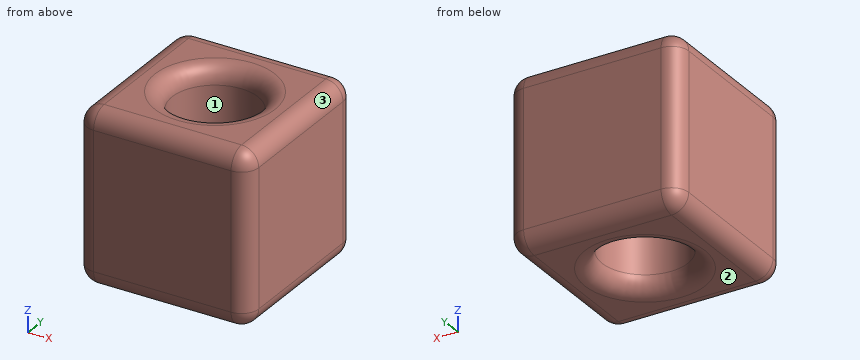
```python
from build123d import *

# Parameters (mm, degrees)
SKETCH2_W           = 100
SKETCH2_H           = 100
BOSS_EXTRUDE1_DEPTH = 100
SKETCH3_R           = 25
CUT_EXTRUDE1_DEPTH  = 100
FILLET1_R           = 10
FILLET2_R           = 10
FILLET3_R           = 10
FILLET4_R           = 10


with BuildPart() as part:
    # Sketch2 → Boss-Extrude1 (new body)
    with BuildSketch(Plane(origin=(0, 0, 0), x_dir=(1, 0, 0), z_dir=(0, 1, 0))):
        with Locations((50, 50)):
            Rectangle(SKETCH2_W, SKETCH2_H)
    extrude(amount=BOSS_EXTRUDE1_DEPTH)

    # Sketch3 → Cut-Extrude1 (cut)
    with BuildSketch(Plane.XY):
        with Locations((50, 50)):
            Circle(SKETCH3_R)
    extrude(amount=-CUT_EXTRUDE1_DEPTH, mode=Mode.SUBTRACT)

    # Fillet1
    fillet1_edges = [part.edges().sort_by_distance(p)[0] for p in [
        (25, 50, 0),
        (50, 0, 0),
        (100, 50, 0),
        (0, 50, 0),
        (50, 100, 0),
    ]]
    fillet(fillet1_edges, radius=FILLET1_R)

    # Fillet2
    fillet2_edges = [part.edges().sort_by_distance(p)[0] for p in [
        (25, 50, -100),
        (50, 100, -100),
        (50, 0, -100),
        (0, 50, -100),
        (100, 50, -100),
    ]]
    fillet(fillet2_edges, radius=FILLET2_R)

    # Fillet3
    # the kernel refuses this fillet: 10 mm, written as the material it takes off along each edge
    with BuildSketch(Plane(origin=(90, 90, -10), x_dir=(1, 0, 0), z_dir=(0, 1, 0))) as fillet3_piece_1_section:
        Polygon((0, 0), (FILLET3_R, 0), (FILLET3_R, -FILLET3_R), (0, -FILLET3_R), align=None)
    fillet3_piece_1 = extrude(amount=FILLET3_R, mode=Mode.PRIVATE)
    fillet3_piece_1 = fillet3_piece_1 - Plane(origin=(90, 90, -10), x_dir=(-0.7071067811865475, 0, -0.7071067811865475), z_dir=(0, 1, 0)) * Sphere(FILLET3_R, mode=Mode.PRIVATE)
    add(fillet3_piece_1, mode=Mode.SUBTRACT)
    with BuildSketch(Plane(origin=(90, 10, -10), x_dir=(0, -1, 0), z_dir=(1, 0, 0))) as fillet3_piece_2_section:
        Polygon((0, 0), (FILLET3_R, 0), (FILLET3_R, -FILLET3_R), (0, -FILLET3_R), align=None)
    fillet3_piece_2 = extrude(amount=FILLET3_R, mode=Mode.PRIVATE)
    fillet3_piece_2 = fillet3_piece_2 - Plane(origin=(90, 10, -10), x_dir=(0, 0.7071067811865475, -0.7071067811865475), z_dir=(1, 0, 0)) * Sphere(FILLET3_R, mode=Mode.PRIVATE)
    add(fillet3_piece_2, mode=Mode.SUBTRACT)
    with BuildSketch(Plane(origin=(90, 90, -90), x_dir=(1, 0, 0), z_dir=(0, 1, 0))) as fillet3_piece_3_section:
        Polygon((0, 0), (FILLET3_R, 0), (FILLET3_R, FILLET3_R), (0, FILLET3_R), align=None)
    fillet3_piece_3 = extrude(amount=FILLET3_R, mode=Mode.PRIVATE)
    fillet3_piece_3 = fillet3_piece_3 - Plane(origin=(90, 90, -90), x_dir=(-0.7071067811865475, 0, 0.7071067811865475), z_dir=(0, 1, 0)) * Sphere(FILLET3_R, mode=Mode.PRIVATE)
    add(fillet3_piece_3, mode=Mode.SUBTRACT)
    with BuildSketch(Plane(origin=(90, 10, -90), x_dir=(0, -1, 0), z_dir=(1, 0, 0))) as fillet3_piece_4_section:
        Polygon((0, 0), (FILLET3_R, 0), (FILLET3_R, FILLET3_R), (0, FILLET3_R), align=None)
    fillet3_piece_4 = extrude(amount=FILLET3_R, mode=Mode.PRIVATE)
    fillet3_piece_4 = fillet3_piece_4 - Plane(origin=(90, 10, -90), x_dir=(0, 0.7071067811865475, 0.7071067811865475), z_dir=(1, 0, 0)) * Sphere(FILLET3_R, mode=Mode.PRIVATE)
    add(fillet3_piece_4, mode=Mode.SUBTRACT)
    with BuildSketch(Plane(origin=(100, 100, -10), x_dir=(-1, 0, 0), z_dir=(0, 0, -1)), Plane(origin=(100, 0, -10), x_dir=(0, 1, 0), z_dir=(0, 0, -1))) as fillet3_piece_5:
        with BuildLine():
            CenterArc((FILLET3_R, -FILLET3_R), FILLET3_R, 90, 90)
            Line((0, -FILLET3_R), (0, 0))
            Line((0, 0), (FILLET3_R, 0))
        make_face()
    extrude(amount=80, mode=Mode.SUBTRACT)

    # Fillet4
    # the kernel refuses this fillet: 10 mm, written as the material it takes off along each edge
    with BuildSketch(Plane(origin=(10, 90, -10), x_dir=(-1, 0, 0), z_dir=(0, 1, 0))) as fillet4_piece_1_section:
        Polygon((0, 0), (FILLET4_R, 0), (FILLET4_R, FILLET4_R), (0, FILLET4_R), align=None)
    fillet4_piece_1 = extrude(amount=FILLET4_R, mode=Mode.PRIVATE)
    fillet4_piece_1 = fillet4_piece_1 - Plane(origin=(10, 90, -10), x_dir=(0.7071067811865475, 0, -0.7071067811865475), z_dir=(0, 1, 0)) * Sphere(FILLET4_R, mode=Mode.PRIVATE)
    add(fillet4_piece_1, mode=Mode.SUBTRACT)
    with BuildSketch(Plane(origin=(10, 10, -10), x_dir=(0, -1, 0), z_dir=(-1, 0, 0))) as fillet4_piece_2_section:
        Polygon((0, 0), (FILLET4_R, 0), (FILLET4_R, FILLET4_R), (0, FILLET4_R), align=None)
    fillet4_piece_2 = extrude(amount=FILLET4_R, mode=Mode.PRIVATE)
    fillet4_piece_2 = fillet4_piece_2 - Plane(origin=(10, 10, -10), x_dir=(0, 0.7071067811865475, -0.7071067811865475), z_dir=(-1, 0, 0)) * Sphere(FILLET4_R, mode=Mode.PRIVATE)
    add(fillet4_piece_2, mode=Mode.SUBTRACT)
    with BuildSketch(Plane(origin=(10, 90, -90), x_dir=(-1, 0, 0), z_dir=(0, 1, 0))) as fillet4_piece_3_section:
        Polygon((0, 0), (FILLET4_R, 0), (FILLET4_R, -FILLET4_R), (0, -FILLET4_R), align=None)
    fillet4_piece_3 = extrude(amount=FILLET4_R, mode=Mode.PRIVATE)
    fillet4_piece_3 = fillet4_piece_3 - Plane(origin=(10, 90, -90), x_dir=(0.7071067811865475, 0, 0.7071067811865475), z_dir=(0, 1, 0)) * Sphere(FILLET4_R, mode=Mode.PRIVATE)
    add(fillet4_piece_3, mode=Mode.SUBTRACT)
    with BuildSketch(Plane(origin=(10, 10, -90), x_dir=(0, -1, 0), z_dir=(-1, 0, 0))) as fillet4_piece_4_section:
        Polygon((0, 0), (FILLET4_R, 0), (FILLET4_R, -FILLET4_R), (0, -FILLET4_R), align=None)
    fillet4_piece_4 = extrude(amount=FILLET4_R, mode=Mode.PRIVATE)
    fillet4_piece_4 = fillet4_piece_4 - Plane(origin=(10, 10, -90), x_dir=(0, 0.7071067811865475, 0.7071067811865475), z_dir=(-1, 0, 0)) * Sphere(FILLET4_R, mode=Mode.PRIVATE)
    add(fillet4_piece_4, mode=Mode.SUBTRACT)
    with BuildSketch(Plane(origin=(0, 100, -90), x_dir=(1, 0, 0), z_dir=(0, 0, 1)), Plane(origin=(0, 0, -90), x_dir=(0, 1, 0), z_dir=(0, 0, 1))) as fillet4_piece_5:
        with BuildLine():
            CenterArc((FILLET4_R, -FILLET4_R), FILLET4_R, 90, 90)
            Line((0, -FILLET4_R), (0, 0))
            Line((0, 0), (FILLET4_R, 0))
        make_face()
    extrude(amount=80, mode=Mode.SUBTRACT)


solid = part.part
```
Build history of the part. All positions in model axes, mm. Face numbers are marked on the shaded views. Round coordinates to 2 decimals unless told otherwise and drop trailing zeros. Write each loop counter-clockwise with the first axis right and the second up, starting at its lowest first coordinate (ties: lowest second). Pieces come first, ordered by that corner, then holes. Notation, with made-up numbers: (41, 12.5) - (77, 12.5) arc R26 cw to (77, 44.5) - close; hole circle Ø5 at (74.5, 47.5). An arc over 180 degrees is marked (long way). Write each question's results on one line, items separated by ' | '. Start each with the question number.
Item 1: Mould opens along X. For the marked faces 1, 2 and 3 say: pulls with the +X half, pulls with the -X half, needs draft (parallel to the pull), parting line crosses it, or undercut.
Item 2: Saw through at D-D (z = -92). Write the cut outline in (x, y).
Item 3: Saw through at A-A (y = 50). Write the cut outline in (x, z), and give its area (3 significant figures).
Item 4: Saw through at C-C (z = -26.5). Write the cut outline in (x, y), and give its area (3 significant figures).
Item 5: Wall check: L1, parallel to Y at x = 50, z = -57; L2, parallel to Y at x = 44.5, z = -22; L3, parallel to Z at x = 9.5, y = 81.5. Give the ranges that are in metal, low to high. Write a range as [from, to].
Item 6: Drop flat-ended pins along their axis: P1, Ø10, axis at x = 70, z = -23, coming from the -Y side; P2, Ø1, axis at x = 48.5, y = 82.5, coming from the +Z side. Give the stop position or say it passes through.
Results are:
1) face 1: undercut | face 2: needs draft | face 3: pulls with the +X half
2) outline: (0.2, 10) arc R9.8 ccw to (10, 0.2) - (90, 0.2) arc R9.8 ccw to (99.8, 10) - (99.8, 90) arc R9.8 ccw to (90, 99.8) - (10, 99.8) arc R9.8 ccw to (0.2, 90) - close; hole circle Ø50.4 at (50, 50)
3) outline: (0, -90) arc R10 ccw to (10, -100) - (15, -100) arc R10 ccw to (25, -90) - (25, -10) arc R10 ccw to (15, 0) - (10, 0) arc R10 ccw to (0, -10) - close; (75, -90) arc R10 ccw to (85, -100) - (90, -100) arc R10 ccw to (100, -90) - (100, -10) arc R10 ccw to (90, 0) - (85, 0) arc R10 ccw to (75, -10) - close | area: 4,830 mm²
4) outline: (0, 10) arc R10 ccw to (10, 0) - (90, 0) arc R10 ccw to (100, 10) - (100, 90) arc R10 ccw to (90, 100) - (10, 100) arc R10 ccw to (0, 90) - close; hole circle Ø50 at (50, 50) | area: 7,950 mm²
5) L1: y = [0, 25], [75, 100] | L2: y = [0, 25.61], [74.39, 100] | L3: z = [-99.99, -0.01]
6) P1: stops at y = 0 | P2: stops at z = -0.2
